Here's how the part is built. I have some questions about the finished solid (model axes, mm). Face numbers are marked on the shaded views. A direction names the side the tool comes from. Round coordinates to 2 decimals unless told otherwise and drop trailing zeros. Write each loop counter-clockwise with the first axis right and the second up, starting at its lowest first coordinate (ties: lowest second). Pieces come first, ordered by that corner, then holes. Notation, with made-up numbers: (-8, 60) - (4, 60) arc R20 cw to (4, 74) - close; hole circle Ø2 at (65, 20.5). An arc over 180 degrees is marked (long way). Write item = value, one per line. Start each with the question number.
Item 1: If we section it at B-B (y = 10): Please give me the cut outline in (x, z), and give its area (3 significant figures).
Item 2: If we section it at C-C (y = -47.5): Please give me the cut outline in (x, z).
Item 3: If we section it at A-A (x = 15.5): Please give me the cut outline in (y, z), and give its area (3 significant figures).
Item 4: For P1, Ø4, axis at x = -82.5, y = -10, coming from the -Z side; P2, Ø1, axis at y = -24.5, z = 9, coming from the -X side; P3, Ø7.5, axis at y = -4.5, z = 8.5, coming from the +X side, each with a flat end and sliding along its axis, tell me the tip position at first contact or that it passes through.
Item 5: If we section it at D-D (x = -82.5): Please give me the cut outline in (y, z).
Item 6: Which directions (+Z, -Z, +X, -X, +Y, -Y) give clear straight access to the entire face, cutting with the end or side of a thin tool? Please do the marked faces 1, 2 and 3.
Item 7: If I drill on line 1 along Y through (x, z) = (-67.5, 13.9); line 2 along Y through (x, z) = (15.5, 0.4); line 3 along X through (y, z) = (-15, 1.25), over which ranges is the centre line in solid material (lowest first)? Write a range as [from, to].
Autodesk Inventor part; units mm, degrees
ref_plane "YZ Plane" through (0, 0, 0) normal (1, 0, 0) x (0, 1, 0)
ref_plane "XZ Plane" through (0, 0, 0) normal (0, 1, 0) x (-1, 0, 0)
ref_plane "XY Plane" through (0, 0, 0) normal (0, 0, 1) x (1, 0, 0)
sketch "スケッチ1" plane through (0, 0, 0) normal (0, 0, 1) x (1, 0, 0)
  line L0 (25.5, -25) -> (-25.5, -25)
  line L1 (-25.5, -25) -> (-25.5, 25)
  line L2 (-25.5, 25) -> (25.5, 25)
  line L3 (25.5, 25) -> (25.5, -25)
  line L4 (25.5, -25) -> (-25.5, 25) construction
  line L5 (-25.5, -25) -> (25.5, 25) construction
  point P0 (0, 0)
  dimension "d0" = 51
  dimension "d1" = 50
extrude "プレート1" add sketch "スケッチ1" along normal blind 2
sketch "スケッチ2" plane through (-23.5, -25, 0) normal (-1, 0, 0) x (0, -1, 0)
  line L0 (-50, 0) -> (0, 0)
  line L1 (0, 0) -> (0, 15)
  line L2 (0, 15) -> (-50, 15)
  line L3 (-50, 15) -> (-50, 0)
edge flange "フランジ1" height 15 angle 90 thickness 2 bend radius 2 thickness toward (-1, 0, 0) relief tear relief width 2 relief depth 1 edges at (-25.5, 0, 2) wall of the first edge with corners at (-23.5, 25, 0) (-23.5, -25, 0) (-23.5, -25, 15) (-23.5, 25, 15)
bend "曲げ1"
corner "コーナー1"
sketch "スケッチ3" plane through (-23.5, 25, 13) normal (0, 0, 1) x (1, 0, 0)
  line L0 (0, -50) -> (0, 0)
  line L1 (0, 0) -> (-71, 0)
  line L2 (-71, 0) -> (-71, -50)
  line L3 (-71, -50) -> (0, -50)
edge flange "フランジ2" height 71 angle 90 thickness 2 bend radius 2 thickness toward (0, 0, 1) relief tear relief width 2 relief depth 1 edges at (-25.5, 0, 15) wall of the first edge with corners at (-23.5, -25, 13) (-23.5, 25, 13) (-94.5, 25, 13) (-94.5, -25, 13)
bend "曲げ2"
corner "コーナー2"
sketch "スケッチ4" plane through (0, 0, 2) normal (0, 0, 1) x (1, 0, 0)
  line L0 (-11.5, -15) -> (15.5, -15)
  line L1 (15.5, -15) -> (15.5, 15)
  line L2 (15.5, 15) -> (-11.5, 15)
  line L3 (-11.5, 15) -> (-11.5, -15)
  line L4 (-11.5, -15) -> (15.5, 15) construction
  line L5 (15.5, -15) -> (-11.5, 15) construction
  line L6 (-21.5, 25) -> (25.5, 25)
  line L7 (25.5, 25) -> (25.5, -25)
  point P0 (0, 0)
  point P1 (2, 0)
  dimension "d23" = 27
  dimension "d25" = 30
  dimension "d26" = 10
  dimension "d27" = 10
hole "穴1" at (-11.5, 15, 2) at (-11.5, -15, 2) at (15.5, -15, 2) at (15.5, 15, 2) direction (0, 0, -1) diameter 5.3 depth 2 tip angle 118
fillet "フィレット1" radius 2 3 edges at (25.5, 25, 1) (25.5, -25, 1) (-94.5, 25, 14)
sketch "スケッチ5" plane through (-27.5, -25, 15) normal (0, 0, 1) x (1, 0, 0)
  line L0 (0, 0) -> (-67, 0)
  line L1 (0, 0) -> (0, 50)
  line L2 (-65, 50) -> (0, 50)
  arc A0 (-65, 50) -> (-67, 48) centre (-65, 48) ccw
  line L3 (-67, 0) -> (-67, 48)
  line L4 (-55, 15) -> (-40, 15)
  line L5 (-40, 15) -> (-40, 35)
  line L6 (-40, 35) -> (-55, 35)
  line L7 (-55, 35) -> (-55, 15)
  line L8 (-55, 15) -> (-40, 35) construction
  line L9 (-40, 15) -> (-55, 35) construction
  point P0 (27.5, 25)
  point P1 (-47.5, 25)
  dimension "d36" = 15
  dimension "d37" = 19.5
  dimension "d38" = 20
  dimension "d39" = 15
hole "穴2" at (-82.5, 10, 15) at (-82.5, -10, 15) at (-67.5, -10, 15) at (-67.5, 10, 15) direction (0, 0, -1) diameter 3.242 depth 11.8 tip angle 118
sketch "スケッチ6" plane through (-94.5, -25, 15) normal (0, 0, 1) x (1, 0, 0)
  circle A0 centre (27, 15) radius 1.621
  circle A1 centre (12, 35) radius 1.621
  circle A2 centre (12, 15) radius 1.621
  circle A3 centre (27, 35) radius 1.621
  arc A4 (2, 50) -> (0, 48) centre (2, 48) ccw
  line L0 (0, 0) -> (0, 48)
  line L1 (67, 0) -> (0, 0)
  line L2 (67, 0) -> (67, 50)
  line L3 (2, 50) -> (67, 50)
  line L4 (0, 0) -> (39, 0)
  line L5 (39, 0) -> (39, -30)
  line L6 (39, -30) -> (0, -30)
  line L7 (0, -30) -> (0, 0)
  point P0 (94.5, 25)
  point P1 (39, 0)
  dimension "d47" = 39
  dimension "d48" = 80
extrude "押し出し1" add sketch "スケッチ6" against normal up to surface (2 mm away) contours L1 L5 L6 L7
chamfer "面取り1" distance 20 angle 45 1 edges at (-55.5, -25, 14)
fillet "フィレット2" radius 2 4 edges at (-94.5, -55, 14) (-55.5, -55, 14) (-55.5, -45, 14) (-35.5, -25, 14)
equation "\"d33\" = Thickness"
equation "\"d2\" = Thickness"
equation "\"d3\" = BendReliefWidth"
equation "\"d4\" = BendReliefDepth"
equation "\"d5\" = MinimumRemnant"
equation "\"d6\" = TransitionRadius"
equation "\"d9\" = BendRadius"
equation "\"d10\" = CornerReliefSize"
equation "\"d11\" = GapSize"
equation "\"d12\" = JacobiRadiusSize"
equation "\"d13\" = BendReliefWidth"
equation "\"d14\" = BendReliefDepth"
equation "\"d15\" = MinimumRemnant"
equation "\"d16\" = TransitionRadius"
equation "\"d19\" = BendRadius"
equation "\"d20\" = CornerReliefSize"
equation "\"d21\" = GapSize"
equation "\"d22\" = JacobiRadiusSize"
equation "\"BendRadius\" = Thickness"
equation "\"BendReliefWidth\" = Thickness"
equation "\"BendReliefDepth\" = 0.5 * Thickness"
equation "\"CornerReliefSize\" = 4 * Thickness"
equation "\"MinimumRemnant\" = 2 * Thickness"
equation "\"TransitionRadius\" = BendRadius"
equation "\"JacobiRadiusSize\" = BendRadius"
equation "\"GapSize\" = Thickness"
properties part number "DragChain_Guide_B"
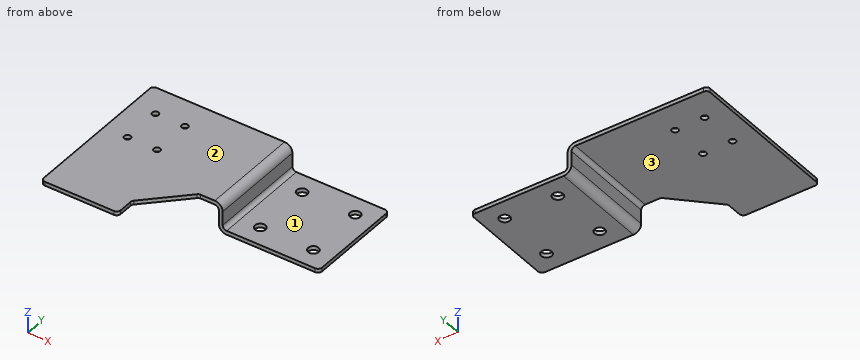
Reply:
q1.outline = (-94.5, 13) - (-84.12, 13) - (-84.12, 15) - (-94.5, 15) - close; (-80.88, 13) - (-69.12, 13) - (-69.12, 15) - (-80.88, 15) - close; (-65.88, 13) - (-27.5, 13) arc R2 cw to (-25.5, 11) - (-25.5, 4) arc R4 ccw to (-21.5, 0) - (25.5, 0) - (25.5, 2) - (-21.5, 2) arc R2 cw to (-23.5, 4) - (-23.5, 11) arc R4 ccw to (-27.5, 15) - (-65.88, 15) - close
q1.area = 248 mm2
q2.outline = (-94.5, 13) - (-55.5, 13) - (-55.5, 15) - (-94.5, 15) - close
q3.outline = (-25, 0) - (-17.65, 0) - (-17.65, 2) - (-25, 2) - close; (-12.35, 0) - (12.35, 0) - (12.35, 2) - (-12.35, 2) - close; (17.65, 0) - (25, 0) - (25, 2) - (17.65, 2) - close
q3.area = 78.8 mm2
q4.P1 = 13
q4.P2 = -25.5
q4.P3 = -23.5
q5.outline = (-55, 13) - (-11.62, 13) - (-11.62, 15) - (-55, 15) - close; (-8.38, 13) - (8.38, 13) - (8.38, 15) - (-8.38, 15) - close; (11.62, 13) - (25, 13) - (25, 15) - (11.62, 15) - close
q6.face_1 = +Z, +X, +Y, -Y
q6.face_2 = +Z, +X, -X, +Y, -Y
q6.face_3 = -Z, -X, +Y, -Y
q7.line_1 = [-55, -11.62], [-8.38, 8.38], [11.62, 25]
q7.line_2 = [-25, -17.65], [-12.35, 12.35], [17.65, 25]
q7.line_3 = [-24.4, -14.15], [-8.85, 12.85], [18.15, 25.5]
